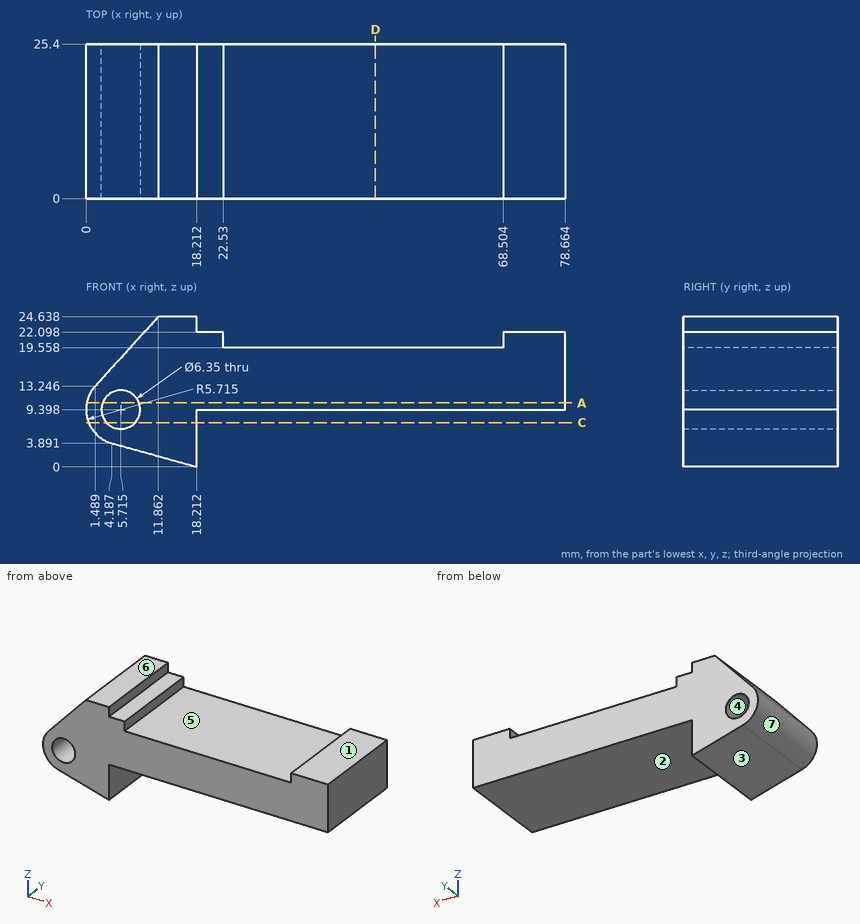
Answer from the drawing. Dimensions are ordinates in mm from the lowest x, y and z of the part. A direction names the side the tool comes from. Give positions to 0.01 mm unless a question says otherwise; leave off trailing zeros. Write each loop counter-clockwise with the first axis right and the second up, starting at its lowest first coordinate (ties: lowest second). Pieces come first, ordered by that corner, then holes. Notation, with made-up numbers: (89, -16.5) -> (115, -16.5) arc R11 cw to (115, -5.5) -> close; hole circle Ø8 at (39.5, 43). An arc over 180 degrees is marked (long way). Use a Markdown table: item, result.
(1) For the marked faces 1, 2 and 3, determine the directions among +Z, -Z, +X, -X, +Y, -Y from which every point of the face is accessible in a straight line to the end or side of a thin tool.
Return value:
| item | result |
|---|---|
| face 1 | +Z, +X, +Y, -Y |
| face 2 | -Z, +X, +Y, -Y |
| face 3 | -Z, -X, +Y, -Y |
(2) Flat-ended cylindrical pins translate along their axes: P1, Ø6, axis at x = 11, y = 9.5, coming from the -Z side; P2, Ø7.5, axis at y = 7, z = 3, coming from the +X side; P3, Ø8, axis at y = 18.5, z = 19, coming from the -X side (1 decimal); P4, Ø5.5, axis at x = 5.715, z = 9.398, coming from the +Y side. Find the tip coordinate at first contact, or state that the pin passes through.
Return value:
| item | result |
|---|---|
| P1 | z = 1.17 |
| P2 | x = 18.21 |
| P3 | x = 3.1 |
| P4 | through |
(3) Section A-A, the plane z = 10.5 is taken. Determine the outline of the cut face in (x, y).
Return value:
| item | result |
|---|---|
| outline | (0.11, 0) -> (2.74, 0) -> (2.74, 25.4) -> (0.11, 25.4) -> close; (8.69, 0) -> (78.66, 0) -> (78.66, 25.4) -> (8.69, 25.4) -> close |
(4) Find the intervals of material crossed by probe 1 along Z at (x, y) = (29.5, 7); probe 2 along X at (y, z) = (16, 7.5) (1 decimal); probe 3 along Z at (x, y) = (5, 9.75) (1 decimal), in increasing order. Write a range as from..to.
Return value:
| item | result |
|---|---|
| probe 1 | 9.4..19.56 |
| probe 2 | 0.3..3.2, 8.3..18.2 |
| probe 3 | 3.7..6.3, 12.5..17.1 |
(5) Section D-D, the plane x = 47.5 is taken. Determine the outline of the cut face in (y, z), then the cut area to 3 significant figures.
Return value:
| item | result |
|---|---|
| outline | (0, 9.4) -> (25.4, 9.4) -> (25.4, 19.56) -> (0, 19.56) -> close |
| area | 258 mm2 |
(6) Determine the mould class of the marked faces 4, 5, 6 and 7 for opening direction X: released by +X, released by -X, zero draft, split by the parting line, or undercut.
Return value:
| item | result |
|---|---|
| face 4 | undercut |
| face 5 | undercut |
| face 6 | zero draft |
| face 7 | released by -X |
(7) Section C-C, the plane z = 7.25 is taken. Determine the outline of the cut face in (x, y), then the cut area to 3 significant figures.
Return value:
| item | result |
|---|---|
| outline | (0.42, 0) -> (3.38, 0) -> (3.38, 25.4) -> (0.42, 25.4) -> close; (8.05, 0) -> (18.21, 0) -> (18.21, 25.4) -> (8.05, 25.4) -> close |
| area | 333 mm2 |
